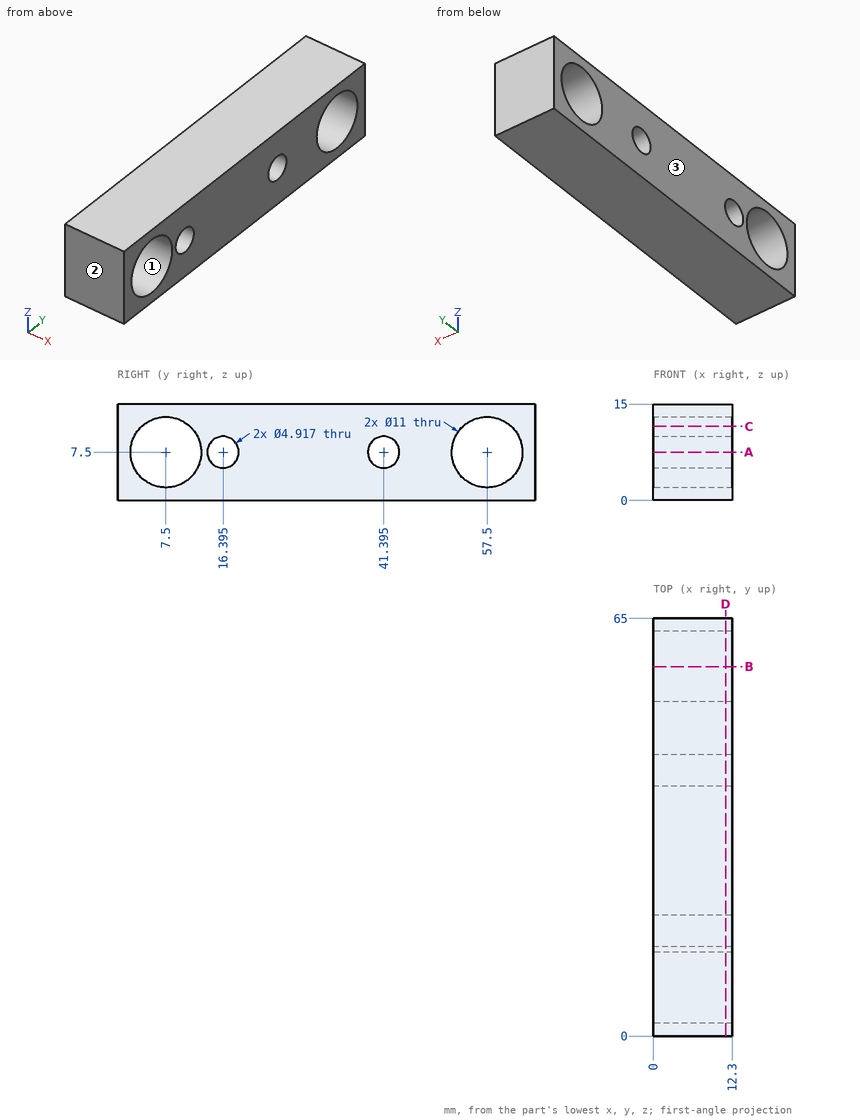
Could you check a few things on this drawing? It's one solid part, dimensions in mm from its lowest x, y, z. Give positions to 0.01 mm unless a question says otherwise; leave off trailing zeros. Order: outer loops, then holes, each group sorted by start corner. A loop starts at its lowest first (then second) coordinate and runs counter-clockwise, first axis right, second up. Notation, with made-up numbers: (69, 18.25) - (119, 18.25) arc R22 ccw to (119, 34.25) - close; hole circle Ø9 at (-10, 88). An arc over 180 degrees is marked (long way). Answer as a JSON object with one key per item and string values. Group by question number.
Item 1: If we section it at D-D on x = 11.25: Please give me the cut outline in (y, z) (1 decimal).
Item 2: If we section it at A-A on z = 7.5: Please give me the cut outline in (x, y), and give its area (3 significant figures).
Item 3: If we mould it in two halves opening along Y, with no side actions, what happens to the marked faces 1, 2 and 3? For each: pulls with the +Y half, pulls with the -Y half, needs draft (parallel to the pull), parting line crosses it, or undercut.
Item 4: If we section it at B-B on y = 57.5: Please give me the cut outline in (x, z).
Item 5: Please list where these lines run through material, in increasing order: probe 1 along Y at (x, z) = (8, 7.5); probe 2 along Y at (x, z) = (9.5, 11); probe 3 along Y at (x, z) = (5, 3.75).
Item 6: If we section it at C-C on z = 11.5: Please give me the cut outline in (x, y), and give its area (3 significant figures).
Result set:
{
 "1": {"outline": "(0, 0) - (65, 0) - (65, 15) - (0, 15) - close; hole circle Ø11 at (7.5, 7.5); hole circle Ø4.9 at (16.4, 7.5); hole circle Ø4.9 at (41.4, 7.5); hole circle Ø11 at (57.5, 7.5)"},
 "2": {"outline": "(0, 0) - (12.3, 0) - (12.3, 2) - (0, 2) - close; (0, 13) - (12.3, 13) - (12.3, 13.94) - (0, 13.94) - close; (0, 18.85) - (12.3, 18.85) - (12.3, 38.94) - (0, 38.94) - close; (0, 43.85) - (12.3, 43.85) - (12.3, 52) - (0, 52) - close; (0, 63) - (12.3, 63) - (12.3, 65) - (0, 65) - close", "area": "408 mm²"},
 "3": {"face 1": "undercut", "face 2": "pulls with the -Y half", "face 3": "needs draft"},
 "4": {"outline": "(0, 0) - (12.3, 0) - (12.3, 2) - (0, 2) - close; (0, 13) - (12.3, 13) - (12.3, 15) - (0, 15) - close"},
 "5": {"probe 1": "0 to 2, 13 to 13.94, 18.85 to 38.94, 43.85 to 52, 63 to 65", "probe 2": "0 to 3.26, 11.74 to 53.26, 61.74 to 65", "probe 3": "0 to 3.48, 11.52 to 53.48, 61.52 to 65"},
 "6": {"outline": "(0, 0) - (12.3, 0) - (12.3, 3.73) - (0, 3.73) - close; (0, 11.27) - (12.3, 11.27) - (12.3, 53.73) - (0, 53.73) - close; (0, 61.27) - (12.3, 61.27) - (12.3, 65) - (0, 65) - close", "area": "614 mm²"}
}
